For this review, take the finished solid that the model builds, in its own axes (mm). A direction names the side the tool comes from. Coordinates: 2 decimals unless noted, no trailing zeros. Loops run counter-clockwise (first coordinate to the right, second up) from the corner with the lowest first, then second, coordinate; pieces in that order, holes last. Notation, with made-up numbers: (-18, -16) -> (5, -16) arc R21 cw to (5, 15) -> close; hole circle Ø3 at (49, 25). An arc over 180 degrees is marked (long way). Answer in a Markdown table with one row per item.
Autodesk Inventor part; units mm, degrees
ref_plane "YZ Plane" through (0, 0, 0) normal (1, 0, 0) x (0, 1, 0)
ref_plane "XZ Plane" through (0, 0, 0) normal (0, 1, 0) x (-1, 0, 0)
ref_plane "XY Plane" through (0, 0, 0) normal (0, 0, 1) x (1, 0, 0)
sketch "Sketch3" plane through (0, 0, 0) normal (0, 0, 1) x (1, 0, 0)
  circle A0 centre (0, 0) radius 3
  dimension "Diameter" = 6
extrude "Extrusion1" add sketch "Sketch3" against normal blind 6
sketch "Sketch4" plane through (0, 0, 0) normal (0, 0, 1) x (1, 0, 0)
  circle A0 centre (0, 0) radius 3
  circle A1 centre (0, 0) radius 5
  dimension "Head_Diameter" = 10
extrude "Extrusion2" add sketch "Sketch4" along normal blind 6 contours A0 | A1
sketch "Sketch5" plane through (0, 0, 6) normal (0, 0, 1) x (1, 0, 0)
  circle A0 centre (0, 0) radius 5
  line L0 (2.8868, 0) -> (1.4434, -2.5)
  line L1 (1.4434, -2.5) -> (-1.4434, -2.5)
  line L2 (-1.4434, -2.5) -> (-2.8868, 0)
  line L3 (-2.8868, 0) -> (-1.4434, 2.5)
  line L4 (-1.4434, 2.5) -> (1.4434, 2.5)
  line L5 (1.4434, 2.5) -> (2.8868, 0)
  line L6 (0, 0) -> (2.8868, 0) construction
  dimension "Hex_Width" = 5
extrude "Extrusion3" cut sketch "Sketch5" against normal blind 3 contours L0 L1 L2 L3 L4 L5
thread "Thread1"
chamfer "Chamfer1" distance 0.6 angle 45 1 edges at (-5, 0, 6)
chamfer "Chamfer2" distance 0.3 angle 45 1 edges at (-3, 0, -6)
equation "\"d14\" = 0.5 * Chamfer"
properties part number "SCREW, SOCKET HD, P, 12.9, M6X1" material "Steel, MS"
Item 1: For L1, parallel to Z at x = -2.5, y = 2.25; L2, parallel to X at y = 2, z = 5.25; L3, parallel to X at y = 2.25, z = 3.5, list the stretches that pass through material, from the lowest coordinate up.
Worked answers:
| item | result |
|---|---|
| L1 | 0 to 6 |
| L2 | -4.58 to -1.73, 1.73 to 4.58 |
| L3 | -4.47 to -1.59, 1.59 to 4.47 |
Item 2: Take a section at A-A, the plane z = 3.75. State the section outline as (x, y) points, and give its area (3 significant figures).
Worked answers:
| item | result |
|---|---|
| outline | circle Ø10 at (0, 0); hole (-2.89, 0) -> (-1.44, -2.5) -> (1.44, -2.5) -> (2.89, 0) -> (1.44, 2.5) -> (-1.44, 2.5) -> close |
| area | 56.9 mm² |
Item 3: Take a section at B-B, the plane x = 0. State the section outline as (y, z) points, and give its area (4 significant figures).
Worked answers:
| item | result |
|---|---|
| outline | (-5, 0) -> (-3, 0) -> (-3, -5.7) -> (-2.7, -6) -> (2.7, -6) -> (3, -5.7) -> (3, 0) -> (5, 0) -> (5, 5.4) -> (4.4, 6) -> (2.5, 6) -> (2.5, 3) -> (-2.5, 3) -> (-2.5, 6) -> (-4.4, 6) -> (-5, 5.4) -> close |
| area | 80.55 mm² |
Item 4: Take a section at C-C, the plane z = 1. State the section outline as (x, y) points.
Worked answers:
| item | result |
|---|---|
| outline | circle Ø10 at (0, 0) |
Item 5: Insertion check: pin 1 (2.5 mm diameter, centred on x = -0.5, z = 4.5, fed in from -Y); pin 2 (5 mm diameter, centred on y = 2.5, z = -4.5, fed in from +X); pin 3 (1 mm diameter, centred on x = -1, z = -4, fed in from +Y); pin 4 (2 mm diameter, centred on x = 4, z = 1.5, fed in from -Y). Each pin has a flat end and moves straight along its axis. Give the tip position at first contact, or say it passes through.
Worked answers:
| item | result |
|---|---|
| pin 1 | y = -5 |
| pin 2 | x = 3 |
| pin 3 | y = 2.96 |
| pin 4 | y = -4 |
Item 6: For faces 5 (the flat face through (3.3, 0.1, 0)), 6 (the flat face through (0, 0, 3)), 7 (the flat face through (0, 0, -6)), list the 3-axis set-ups (+Z, -Z, +X, -X, +Y, -Y) from which the entire face can be reached by the end or side of a thin tool; tool diameter is ignored.
Worked answers:
| item | result |
|---|---|
| face 5 | -Z |
| face 6 | +Z |
| face 7 | -Z, +X, -X, +Y, -Y |
Item 7: The part is to be moulded in two halves that separate along Y. For faces 1 (the flat face through (2, -2, 6)), 2 (the flat face through (2.155, 1.267, 4.521)), 3 (the cylindrical face through (-1.08, 4.88, 2.66)), 4 (the flat face through (-2.175, 1.233, 4.521)), say which applies: +Y half, -Y half, draft (parallel to the pull), parting line (faces both ways), or undercut.
Worked answers:
| item | result |
|---|---|
| face 1 | draft |
| face 2 | undercut |
| face 3 | parting line |
| face 4 | undercut |
Item 8: Take a section at D-D, the plane z = -3.25. State the section outline as (x, y) points, and give its area (3 significant figures).
Worked answers:
| item | result |
|---|---|
| outline | circle Ø6 at (0, 0) |
| area | 28.3 mm² |
